The model under review builds one solid part; all positions refer to its coordinate system, in mm. A direction names the side the tool comes from. Round coordinates to 2 decimals unless told otherwise and drop trailing zeros. Order: outer loops, then holes, each group sorted by start corner. A loop starts at its lowest first (then second) coordinate and runs counter-clockwise, first axis right, second up. Notation, with made-up numbers: M 12.25,64 L 35.25,64 A14 ccw 35.25,80 Z; hole C 28,10 d3. An arc over 180 degrees is marked long. Use a Markdown table: item, result. Add a question column.
1. Consider section A-A on x = 14. State the section outline as (y, z) points, then the cut area to 3 significant figures.
2. Insertion check: P1, Ø3.5, axis at y = 9, z = 9, coming from the +X side; P2, Ø2, axis at y = 20.5, z = 7.5, coming from the +X side; P3, Ø5, axis at x = 16.5, z = 5, coming from the -Y side; P4, Ø11, axis at x = 15, z = 10, coming from the +Y side. Each pin has a flat end and moves straight along its axis. Give the tip position at first contact, or say it passes through.
3. Consider section C-C on y = 27. State the section outline as (x, z) points, then the cut area to 3 significant figures.
4. For faces 1 (the cylindrical face through (13.85, 3.45, -1.93)), 2 (the flat face through (2, 11, -13)), 3 (the flat face through (9, 12, 1.5)), list the 3-axis set-ups (+Z, -Z, +X, -X, +Y, -Y) from which the entire face can be reached by the end or side of a thin tool; tool diameter is ignored.
5. Consider section D-D on x = 20. State the section outline as (y, z) points.
6. The part is to be moulded in two halves that separate along Y. For faces 4 (the flat face through (2, 31, -12)), 5 (the flat face through (3, 17, -7)), 6 (the conical face through (1.406, 7.847, 10.258)), say which applies: +Y half, -Y half, draft (parallel to the pull), parting line (faces both ways), or undercut.
7. Consider section B-B on z = -5. State the section outline as (x, y) points, then the cut area to 3 significant figures.
8. To check wall thickness, follow probe 1 along Z at (x, y) = (0.5, 9); probe 2 along Y at (x, z) = (0.7, -9); probe 3 along X at (y, z) = (1.45, -7.5). State the ranges of each line that lie inside material, in increasing order.
from build123d import *

# Parameters (mm, degrees)
EXTRUDE_1_DEPTH          = 13
SKETCH_4_R               = 1.5
CUT_EXTRUDE_1_DEPTH      = 3
EXTRUDE_2_DEPTH          = 1.5
CHAMFER_1_SIZE           = 2
FILLET_1_R               = 1.5
HOLE_WIZARD_1_AT_2_COUNT = 2
HOLE_WIZARD_1_AT_2_PITCH = 18
HOLE_WIZARD_1_AT_3_COUNT = 2
HOLE_WIZARD_1_AT_3_PITCH = 25.455844123
HOLE_WIZARD_1_AT_4_COUNT = 2
HOLE_WIZARD_1_AT_4_PITCH = 18


with BuildPart() as part:
    # 草图1 → 凸台-拉伸1 (new, symmetric)
    with BuildSketch(Plane.XY):
        Polygon((0, 0), (25, 0), (25, 3), (3, 3), (3, 32), (0, 32), align=None)
    extrude(amount=EXTRUDE_1_DEPTH, both=True)

    # 草图4 → 切除-拉伸1 (cut)
    with BuildSketch(Plane.XZ):
        with Locations(Location((10, -7.5, 0), (0, 0, 270))):
            Circle(SKETCH_4_R)
        with Locations(Location((10, 7.5, 0), (0, 0, 270))):
            Circle(SKETCH_4_R)
        with Locations(Location((20, 8.5, 0), (0, 0, 270))):
            Circle(SKETCH_4_R)
        with Locations(Location((20, -8.5, 0), (0, 0, 270))):
            Circle(SKETCH_4_R)
    extrude(amount=-CUT_EXTRUDE_1_DEPTH, mode=Mode.SUBTRACT)

    # 草图2 → 凸台-拉伸2 (add, symmetric)
    with BuildSketch(Plane.XY):
        Polygon((3, 32), (3, 3), (25, 3), align=None)
    extrude(amount=EXTRUDE_2_DEPTH, both=True)

    # 倒角1
    chamfer_1_edges = [part.edges().sort_by_distance(p)[0] for p in [
        (25, 1.5, 13),
        (1.5, 32, 13),
        (1.5, 32, -13),
        (25, 1.5, -13),
    ]]
    chamfer(chamfer_1_edges, length=CHAMFER_1_SIZE)

    # 圆角1
    # the kernel refuses this fillet: 1.5 mm, written as the material it adds along each edge
    with BuildSketch(Plane(origin=(3, 3, -1.5), x_dir=(0, 0, -1), z_dir=(1, 0, 0))) as fillet_1_piece_1_section:
        with BuildLine():
            CenterArc((FILLET_1_R, FILLET_1_R), FILLET_1_R, 180, 90)
            Line((0, FILLET_1_R), (0, 0))
            Line((0, 0), (FILLET_1_R, 0))
        make_face()
    fillet_1_piece_1 = extrude(amount=25.75, mode=Mode.PRIVATE)
    fillet_1_piece_1 = split(fillet_1_piece_1, bisect_by=Plane(origin=(20.775844012, 8.568205621, -1.836675405), z_dir=(-0.7966912709023963, -0.6043864813742318, 0)), keep=Keep.TOP, mode=Mode.PRIVATE)
    add(fillet_1_piece_1)
    with BuildSketch(Plane(origin=(3, 3, 1.5), x_dir=(0, 0, 1), z_dir=(1, 0, 0))) as fillet_1_piece_2_section:
        with BuildLine():
            CenterArc((FILLET_1_R, -FILLET_1_R), FILLET_1_R, 90, 90)
            Line((0, -FILLET_1_R), (0, 0))
            Line((0, 0), (FILLET_1_R, 0))
        make_face()
    fillet_1_piece_2 = extrude(amount=25.75, mode=Mode.PRIVATE)
    fillet_1_piece_2 = split(fillet_1_piece_2, bisect_by=Plane(origin=(20.775844012, 8.568205621, 1.836675405), z_dir=(-0.7966912709023963, -0.6043864813742318, 0)), keep=Keep.TOP, mode=Mode.PRIVATE)
    add(fillet_1_piece_2)

    # 草图6 → 打孔尺寸(%根据)开槽半沉头木螺钉的类型1 (revolve, cut)
    with BuildSketch(Plane(origin=(3, 9, -9), x_dir=(0, 0, -1), z_dir=(0, 1, 0))):
        Polygon((0, 0), (0, 3), (1.6, 3), (1.6, 1.7), (3.3, 0), align=None)
    hole_wizard_1 = revolve(axis=Axis((9.35, 9, -9), (-1, 0, 0)), mode=Mode.SUBTRACT)

    # 打孔尺寸(%根据)开槽半沉头木螺钉的类型1 at 2: 打孔尺寸(%根据)开槽半沉头木螺钉的类型1 ×2
    with Locations(*[(0, 0, i * HOLE_WIZARD_1_AT_2_PITCH) for i in range(1, HOLE_WIZARD_1_AT_2_COUNT)]):
        add(hole_wizard_1, mode=Mode.SUBTRACT)

    # 打孔尺寸(%根据)开槽半沉头木螺钉的类型1 at 3: 打孔尺寸(%根据)开槽半沉头木螺钉的类型1 ×2
    with Locations(*[Vector(0, 0.7071067811865476, 0.7071067811865476) * (i * HOLE_WIZARD_1_AT_3_PITCH) for i in range(1, HOLE_WIZARD_1_AT_3_COUNT)]):
        add(hole_wizard_1, mode=Mode.SUBTRACT)

    # 打孔尺寸(%根据)开槽半沉头木螺钉的类型1 at 4: 打孔尺寸(%根据)开槽半沉头木螺钉的类型1 ×2
    with Locations(*[(0, i * HOLE_WIZARD_1_AT_4_PITCH, 0) for i in range(1, HOLE_WIZARD_1_AT_4_COUNT)]):
        add(hole_wizard_1, mode=Mode.SUBTRACT)


solid = part.part
Answer block:
| question | item | result |
|---|---|---|
| 1 | outline | M 0,-13 L 3,-13 L 3,-3 A1.5 cw 4.5,-1.5 L 17.5,-1.5 L 17.5,1.5 L 4.5,1.5 A1.5 cw 3,3 L 3,13 L 0,13 Z |
| 1 | area | 122 mm^2 |
| 2 | P1 | x = 1.45 |
| 2 | P2 | x = 3 |
| 2 | P3 | y = 0 |
| 2 | P4 | y = 3 |
| 3 | outline | M 0,-13 L 3,-13 L 3,-12.3 L 1.3,-10.6 L 0,-10.6 Z; M 0,-7.4 L 1.3,-7.4 L 3,-5.7 L 3,-1.5 L 6.79,-1.5 L 6.79,1.5 L 3,1.5 L 3,5.7 L 1.3,7.4 L 0,7.4 Z; M 0,10.6 L 1.3,10.6 L 3,12.3 L 3,13 L 0,13 Z |
| 3 | area | 64.4 mm^2 |
| 4 | face 1 | -Z, +X, +Y |
| 4 | face 2 | -Z, +X, -X, +Y, -Y |
| 4 | face 3 | +Z, +X, +Y |
| 5 | outline | M 0,-13 L 3,-13 L 3,-10 L 0,-10 Z; M 0,-7 L 3,-7 L 3,-3 A1.5 cw 4.5,-1.5 L 9.59,-1.5 L 9.59,1.5 L 4.5,1.5 A1.5 cw 3,3 L 3,7 L 0,7 Z; M 0,10 L 3,10 L 3,13 L 0,13 Z |
| 6 | face 4 | +Y half |
| 6 | face 5 | draft |
| 6 | face 6 | undercut |
| 7 | outline | M 0,0 L 25,0 L 25,3 L 3,3 L 3,32 L 0,32 Z |
| 7 | area | 162 mm^2 |
| 8 | probe 1 | -13 to -10.6, -7.4 to 7.4, 10.6 to 13 |
| 8 | probe 2 | 0 to 7.4, 10.6 to 25.4, 28.6 to 32 |
| 8 | probe 3 | 0 to 8.5, 11.5 to 18.88, 21.12 to 25 |
